from build123d import *

# Parameters (mm, degrees)
SKETCH_1_R             = 7
SKETCH_1_R_2           = 5.5
EXTRUDE_1_DEPTH        = 30
EXTRUDE_START          = -7
SKETCH_2_R             = 15
SKETCH_2_R_2           = 5.5
EXTRUDE_2_DEPTH        = 7
SKETCH_5_W             = 5.5
SKETCH_5_H             = 9
CUT_EXTRUDE_4_DEPTH    = 15
HOLE_WIZARD_M3_1_D     = 2.5
HOLE_WIZARD_M3_1_DEPTH = 9.5
HOLE_WIZARD_M3_1_TIP   = 0.751075774
FILLET_1_R             = 1
SKETCH1_R              = 7.5
EXTRUDE1_DEPTH         = 5
CHAMFER1_SIZE          = 1
SKETCH_9_R             = 18
CUT_EXTRUDE_1_DEPTH    = 55
SKETCH_10_R            = 9
CUT_EXTRUDE_2_DEPTH    = 22.914607001
CHAMFER_5_SIZE         = 1
SKETCH_12_OUTSIDE_W    = 15.516
SKETCH_12_OUTSIDE_H    = 36.016
CUT_EXTRUDE_4_2_DEPTH  = 15


with BuildPart() as part:
    # 草图1 → 拉伸1 (new, symmetric)
    with BuildSketch(Plane.XY):
        Circle(SKETCH_1_R)
        Circle(SKETCH_1_R_2, mode=Mode.SUBTRACT)
    extrude(amount=EXTRUDE_1_DEPTH, both=True)

    # 草图2 → 拉伸2 (add)
    with BuildSketch(Plane.XY.offset(30).offset(EXTRUDE_START)):
        Circle(SKETCH_2_R)
        Circle(SKETCH_2_R_2, mode=Mode.SUBTRACT)
    extrude_2 = extrude(amount=EXTRUDE_2_DEPTH)

    # 镜向1: 拉伸2 across plane
    add(extrude_2.mirror(Plane.XY))

    # 草图5 → Cut-Extrude 4 (cut, symmetric)
    with BuildSketch(Plane(origin=(0, 0, 0), x_dir=(0, 0, -1), z_dir=(1, 0, 0))):
        with Locations((-27.25, -15.5)):
            Rectangle(SKETCH_5_W, SKETCH_5_H)
        with Locations((27.25, -15.5)):
            Rectangle(SKETCH_5_W, SKETCH_5_H)
    extrude(amount=CUT_EXTRUDE_4_DEPTH, both=True, mode=Mode.SUBTRACT)

    # M3 螺纹孔1
    with Locations(Plane(origin=(-8, -11, 27.5), x_dir=(0, 0, -1), z_dir=(0, -1, 0))):
        with Locations((0, 0), (0, 16), (55, 0), (55, 16)):
            Hole(HOLE_WIZARD_M3_1_D / 2, depth=HOLE_WIZARD_M3_1_DEPTH)
            with Locations((0, 0, -(HOLE_WIZARD_M3_1_DEPTH + HOLE_WIZARD_M3_1_TIP / 2))):  # 118° drill point
                Cone(0, HOLE_WIZARD_M3_1_D / 2, HOLE_WIZARD_M3_1_TIP, mode=Mode.SUBTRACT)

    # 圆角1
    fillet_1_edges = [part.edges().sort_by_distance(p)[0] for p in [
        (-7, 0, -23),
        (-7, 0, 23),
    ]]
    fillet(fillet_1_edges, radius=FILLET_1_R)

    # Sketch1 → Extrude1 (cut)
    with BuildSketch(Plane(origin=(0, 0, 30), x_dir=(-1, 0, 0), z_dir=(0, 0, -1))):
        Circle(SKETCH1_R)
    extrude(amount=EXTRUDE1_DEPTH, mode=Mode.SUBTRACT)

    # Chamfer1
    chamfer1_edges = [part.edges().sort_by_distance(p)[0] for p in [
        (-5.5, 0, 25),
    ]]
    chamfer(chamfer1_edges, length=CHAMFER1_SIZE)

    # 草图9 → 切除-拉伸1 (cut)
    with BuildSketch(Plane(origin=(0, 0, -24.5), x_dir=(-1, 0, 0), z_dir=(0, 0, -1))):
        Circle(SKETCH_9_R)
    extrude(amount=-CUT_EXTRUDE_1_DEPTH, mode=Mode.SUBTRACT)

    # 草图10 → 切除-拉伸2 (cut, through all)
    with BuildSketch(Plane(origin=(0, 0, -30), x_dir=(-1, 0, 0), z_dir=(0, 0, -1))):
        Circle(SKETCH_10_R)
    extrude(amount=-CUT_EXTRUDE_2_DEPTH, mode=Mode.SUBTRACT)

    # 倒角5
    chamfer_5_edges = [part.edges().sort_by_distance(p)[0] for p in [
        (9, 0, -24.5),
        (9, 0, -30),
        (0, 15, -30),
        (0, 15, -24.5),
    ]]
    chamfer(chamfer_5_edges, length=CHAMFER_5_SIZE)

    # 草图12 outside → Cut-Extrude 4 2 (cut, symmetric)
    with BuildSketch(Plane(origin=(0, 0, 0), x_dir=(0, 0, -1), z_dir=(1, 0, 0))):
        with Locations((27.25, 2)):
            Rectangle(SKETCH_12_OUTSIDE_W, SKETCH_12_OUTSIDE_H)
        Polygon((26, 14), (30, 10), (30, -11), (22, -11), (22, 14), align=None, mode=Mode.SUBTRACT)
    extrude(amount=CUT_EXTRUDE_4_2_DEPTH, both=True, mode=Mode.SUBTRACT)


solid = part.part
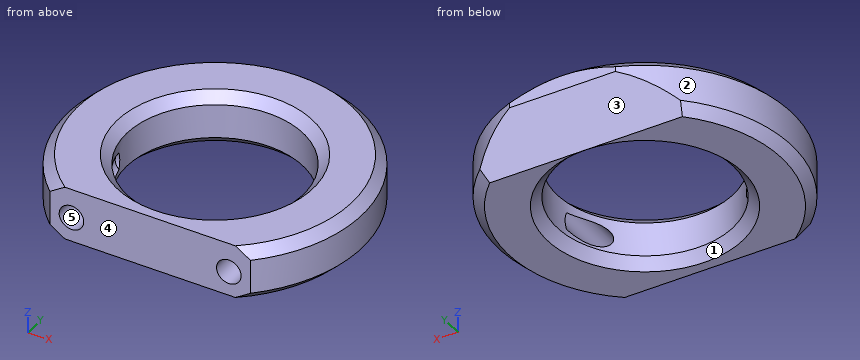
Design review of the part built by this model. Coordinates are the model's own, in mm. Face numbers are marked on the shaded views. A direction names the side the tool comes from. Coordinates: 2 decimals unless noted, no trailing zeros. Write each loop counter-clockwise with the first axis right and the second up, starting at its lowest first coordinate (ties: lowest second). Pieces come first, ordered by that corner, then holes. Notation, with made-up numbers: (-19.5, 8.5) - (-2.5, 8.5) arc R17 cw to (-2.5, 29.5) - close; hole circle Ø2 at (-10.75, 85). An arc over 180 degrees is marked (long way). Use one line per item in the form item = value.
Q1. Consider section C-C (z = -24.95). Write out the cut boundary in (x, y), plus the area to 3 significant figures.
Taken from the geometry:
outline = (-9.37, -11) - (9.37, -11) arc R14.45 ccw to (3.58, 14) - (-3.58, 14) arc R14.45 ccw to start; hole circle Ø19.1 at (0, 0)
area = 323 mm^2
Q2. Consider section B-B (z = -27.5). Write out the cut boundary in (x, y), plus the area to 3 significant figures.
Taken from the geometry:
outline = (-10.2, -11) - (-9.25, -11) - (-9.25, -1.5) - (-8.91, -1.29) arc R9 cw (long way) to (8.91, -1.29) - (9.25, -1.5) - (9.25, -11) - (10.2, -11) arc R15 ccw to (8.29, 12.5) - (-8.29, 12.5) arc R15 ccw to start; (-6.75, -11) - (6.75, -11) - (6.75, -5.95) arc R9 cw to (-6.75, -5.95) - close
area = 332 mm^2
Q3. For probe 1 along Z at (x, y) = (8, -7.5); probe 2 along X at (y, z) = (-6.25, -27.5); probe 3 along X at (y, z) = (-0.25, -27.5), list the stretches that pass through material, from the lowest coordinate up.
Taken from the geometry:
probe_1 = -30 to -28.75, -26.25 to -24.5
probe_2 = -13.64 to -9.25, -6.75 to -6.48, 6.48 to 6.75, 9.25 to 13.64
probe_3 = -15 to -9, 9 to 15
Q4. Consider section D-D (y = -7.25). Count the separate pieces of the cut face and the enclosed holes in it, plus the area to 3 significant figures.
Taken from the geometry:
separate_pieces = 2
enclosed_holes = 2
area = 70.5 mm^2
Q5. The part is to be moulded in two halves that separate along X. For the marked faces 1, 2 and 3, say which applies: +X half, -X half, draft (parallel to the pull), parting line (faces both ways), or undercut.
Taken from the geometry:
face_1 = undercut
face_2 = -X half
face_3 = draft
Q6. Consider section A-A (y = 0). Write out the cut boundary in (x, z), plus the area to 3 significant figures.
Taken from the geometry:
outline = (-15, -29) - (-14, -30) - (-10, -30) - (-9, -29) - (-9, -25.5) - (-10, -24.5) - (-14, -24.5) - (-15, -25.5) - close; (9, -29) - (10, -30) - (14, -30) - (15, -29) - (15, -25.5) - (14, -24.5) - (10, -24.5) - (9, -25.5) - close
area = 62.0 mm^2
Q7. Insertion check: pin 1 Ø3 at (y, z) = (-4, -27.5) entering from -X; pin 2 Ø3 at (x, z) = (-8, -27.5) entering from +Y; pin 3 Ø12 at (x, y) = (4, -8.5) entering from -Z; pin 4 Ø2 at (y, z) = (1.5, -29) entering from -X. Each pin has a flat end and moves straight along its axis. Give the tip position at first contact, or say it passes through.
Taken from the geometry:
pin_1 = -14.79
pin_2 = 13.38
pin_3 = -30
pin_4 = -14.99
Q8. Machinability: for the marked faces 4 and 5, which of the approach directions +Z, -Z, +X, -X, +Y, -Y give a long, thin tool a straight path to every point of the face, cutting with its end or side? Answer none if there is none.
Taken from the geometry:
face_4 = +Z, -Z, +X, -X, -Y
face_5 = -Y
